The listing builds one solid part. Answer for the finished solid, in the listing's coordinates (mm). A direction names the side the tool comes from. Round coordinates to 2 decimals unless told otherwise and drop trailing zeros. Write each loop counter-clockwise with the first axis right and the second up, starting at its lowest first coordinate (ties: lowest second). Pieces come first, ordered by that corner, then holes. Notation, with made-up numbers: (-27.75, 39.25) - (9.25, 39.25) arc R24 cw to (9.25, 50.25) - close; hole circle Ø1 at (-27.5, 54.25). An arc over 180 degrees is marked (long way). Return JSON: item names as keys, results as strings. Group by question number.
(1) Each of these flat-tipped pins is pushed along its axis until it touches: pin 1 (2 mm diameter, centred on x = 13, z = 17, fed in from +Y); pin 2 (3 mm diameter, centred on x = 32, z = 16.5, fed in from -Y); pin 3 (10 mm diameter, centred on x = 24.5, y = -16, fed in from +Z). Where does it stop, or does it pass through?
(2) Determine the mould class of faces 1 (the flat face through (33, -19, 0)), 2 (the flat face through (5.906, -20, 16)), 3 (the flat face through (64.626, -20, 6)) for opening direction X: +X half, -X half, draft (parallel to the pull), parting line (faces both ways), or undercut.
(3) Find the intervals of material crossed by line 1 along Y through (x, z) = (53, 13.75); line 2 along Z through (x, y) = (45, -36); line 3 along Z through (x, y) = (41.5, -5), in increasing order. Write a range as [from, to].
(4) Section B-B, the plane y = -11 is taken. Write down the section's boundary in (x, z), then the cut area to 3 significant figures.
(5) Section D-D, the plane z = 4.25 is taken. Write down the section's boundary in (x, y), then the cut area to 3 significant figures.
(6) Section C-C, the plane x = 52 is taken. Write down the section's boundary in (y, z), then the cut area to 3 significant figures.
(7) Section A-A, the plane z = 11.5 is taken. Write down the section's boundary in (x, y), then the cut area to 3 significant figures.
(8) Which of the six approach directions +Z, -Z, +X, -X, +Y, -Y give full straight-line access (tool end or side, diameter ignored) to faces 4 (the flat face through (32, -32, 19.05)), 5 (the flat face through (33, -4.809, 16)), 6 (the flat face through (33, -33.866, 16)), 7 (the flat face through (58.961, -20, 15)), 8 (the flat face through (33, -19, 2.54))?
```python
from build123d import *

# Parameters (mm, degrees)
F0_W     = 67.1657696366
F0_H     = 38.6754088104
F1_DEPTH = 12.7
F2_W     = 55.595561862
F2_H     = 29.0567195043
F3_DEPTH = 6.35
F4_T     = -2.54


with BuildPart() as f1:
    # F0 (on Top) → F1 (new body)
    with BuildSketch(Plane.XY):
        with Locations((33.5828848183, -19.3377044052)):
            Rectangle(F0_W, F0_H)
    extrude(amount=F1_DEPTH)

    # F2 (on face) → F3 (join)
    with BuildSketch(Plane.XY.offset(12.7)):
        with Locations((33.7035246193, -19.3377044052)):
            Rectangle(F2_W, F2_H)
    extrude(amount=F3_DEPTH)

    # F4
    f4_openings = [f1.faces().sort_by_distance(p)[0] for p in [
        (33.703525, -19.337704, 19.05),
    ]]
    offset(amount=F4_T, openings=f4_openings, kind=Kind.INTERSECTION)


solid = f1.part
```
Working result:
{
 "1": {"pin 1": "stops at y = -4.81", "pin 2": "stops at y = -33.87", "pin 3": "stops at z = 2.54"},
 "2": {"face 1": "draft", "face 2": "-X half", "face 3": "undercut"},
 "3": {"line 1": "y = [-33.87, -31.33], [-7.35, -4.81]", "line 2": "z = [0, 2.54], [10.16, 12.7]", "line 3": "z = [0, 2.54], [10.16, 19.05]"},
 "4": {"outline": "(0, 0) - (67.17, 0) - (67.17, 12.7) - (61.5, 12.7) - (61.5, 19.05) - (58.96, 19.05) - (58.96, 10.16) - (64.63, 10.16) - (64.63, 2.54) - (2.54, 2.54) - (2.54, 10.16) - (8.45, 10.16) - (8.45, 19.05) - (5.91, 19.05) - (5.91, 12.7) - (0, 12.7) - close", "area": "284 mm^2"},
 "5": {"outline": "(0, -38.68) - (67.17, -38.68) - (67.17, 0) - (0, 0) - close; hole (2.54, -36.14) - (64.63, -36.14) - (64.63, -2.54) - (2.54, -2.54) - close", "area": "512 mm^2"},
 "6": {"outline": "(-38.68, 0) - (0, 0) - (0, 12.7) - (-4.81, 12.7) - (-4.81, 19.05) - (-7.35, 19.05) - (-7.35, 10.16) - (-2.54, 10.16) - (-2.54, 2.54) - (-36.14, 2.54) - (-36.14, 10.16) - (-31.33, 10.16) - (-31.33, 19.05) - (-33.87, 19.05) - (-33.87, 12.7) - (-38.68, 12.7) - close", "area": "207 mm^2"},
 "7": {"outline": "(0, -38.68) - (67.17, -38.68) - (67.17, 0) - (0, 0) - close; hole (8.45, -31.33) - (58.96, -31.33) - (58.96, -7.35) - (8.45, -7.35) - close", "area": "1,390 mm^2"},
 "8": {"face 4": "+Z, +X, -X, +Y, -Y", "face 5": "+Z, +X, -X, +Y", "face 6": "+Z, +X, -X, -Y", "face 7": "+Z", "face 8": "none"}
}
